```python
from build123d import *

# Parameters (mm, degrees)
F0_R     = 6.35
F1_DEPTH = 3.175


with BuildPart() as f1:
    # F0 (on Front) → F1 (new body, symmetric)
    with BuildSketch(Plane.XZ):
        with BuildLine():
            ThreePointArc((-17.4334869568, 77.4671706545), (-21.0250628511, 76.5704625087), (-24.5709427988, 75.5073358467))
            ThreePointArc((-24.5709427988, 75.5073358467), (-28.0634202853, 74.2801012289), (-31.4949046301, 72.8914259638))
            ThreePointArc((-31.4949046301, 72.8914259638), (-29.5170408255, 62.9143726492), (-19.6585851248, 60.4114964503))
            ThreePointArc((-19.6585851248, 60.4114964503), (-14.8988685075, 63.8720589464), (-13.081, 69.469))
            ThreePointArc((-13.081, 69.469), (-14.2395846465, 74.0218803116), (-17.4334869568, 77.4671706545))
        make_face()
        with BuildLine():
            ThreePointArc((-24.5709427988, 75.5073358467), (-18.8747057723, 74.6070875222), (-16.256, 69.469))
            ThreePointArc((-16.256, 69.469), (-26.3372942277, 64.3309124778), (-24.5709427988, 75.5073358467))
        make_face(mode=Mode.SUBTRACT)
        with BuildLine():
            ThreePointArc((-31.4949046301, 72.8914259638), (-28.0634202853, 74.2801012289), (-24.5709427988, 75.5073358467))
            ThreePointArc((-24.5709427988, 75.5073358467), (-21.0250628511, 76.5704625087), (-17.4334869568, 77.4671706545))
            ThreePointArc((-17.4334869568, 77.4671706545), (-25.5534143712, 78.5265037137), (-31.4949046301, 72.8914259638))
        make_face()
        with BuildLine():
            ThreePointArc((59.6305906851, 52.4335927744), (24.5319973939, 75.5199980174), (-17.4334869568, 77.4671706545))
            ThreePointArc((-17.4334869568, 77.4671706545), (-14.2395846465, 74.0218803116), (-13.081, 69.469))
            ThreePointArc((-13.081, 69.469), (-14.8988685075, 63.8720589464), (-19.6585851248, 60.4114964503))
            ThreePointArc((-19.6585851248, 60.4114964503), (19.192650723, 60.561134655), (50.8659607408, 38.0613046332))
            ThreePointArc((50.8659607408, 38.0613046332), (50.9228529034, 47.8852145144), (59.6305906851, 52.4335927744))
        make_face()
        with BuildLine():
            ThreePointArc((-19.6585851248, 60.4114964503), (-29.5170408255, 62.9143726492), (-31.4949046301, 72.8914259638))
            ThreePointArc((-31.4949046301, 72.8914259638), (-62.5829136435, 48.8719542947), (-78.3514836066, 12.8892984033))
            ThreePointArc((-78.3514836066, 12.8892984033), (-68.4945244609, 13.5260066408), (-63.373, 5.08))
            ThreePointArc((-63.373, 5.08), (-69.0923257109, -3.6516933183), (-79.3819172084, -1.8974237821))
            ThreePointArc((-79.3819172084, -1.8974237821), (-67.3022929991, -42.1365678923), (-36.3814305576, -70.5796040459))
            ThreePointArc((-36.3814305576, -70.5796040459), (-34.1498428756, -61.0672736312), (-24.7158919074, -58.5246406199))
            ThreePointArc((-24.7158919074, -58.5246406199), (-63.4722358852, 2.6989153756), (-19.6585851248, 60.4114964503))
        make_face()
        with BuildLine():
            ThreePointArc((68.58, 42.926), (65.9907092743, 49.4545191171), (59.6305906851, 52.4335927744))
            ThreePointArc((59.6305906851, 52.4335927744), (64.2293016822, 46.6871053087), (68.276185728, 40.5395049195))
            ThreePointArc((68.276185728, 40.5395049195), (68.5037411611, 41.7231220052), (68.58, 42.926))
        make_face()
        with BuildLine():
            ThreePointArc((68.276185728, 40.5395049195), (64.2293016822, 46.6871053087), (59.6305906851, 52.4335927744))
            ThreePointArc((59.6305906851, 52.4335927744), (50.9228529034, 47.8852145144), (50.8659607408, 38.0613046332))
            ThreePointArc((50.8659607408, 38.0613046332), (51.3882284212, 37.3531638847), (51.9006383071, 36.6378576855))
            ThreePointArc((51.9006383071, 36.6378576855), (61.2626352015, 33.6603660866), (68.276185728, 40.5395049195))
        make_face()
        with Locations((59.055, 42.926)):
            Circle(F0_R, mode=Mode.SUBTRACT)
        with BuildLine():
            ThreePointArc((-63.373, 5.08), (-68.4945244609, 13.5260066408), (-78.3514836066, 12.8892984033))
            ThreePointArc((-78.3514836066, 12.8892984033), (-78.8370586265, 9.4766652265), (-79.1740663586, 6.0461734122))
            ThreePointArc((-79.1740663586, 6.0461734122), (-72.4135009686, 11.4114896106), (-66.548, 5.08))
            ThreePointArc((-66.548, 5.08), (-72.8548244643, -1.2698532167), (-79.2474128734, 4.9936509246))
            ThreePointArc((-79.2474128734, 4.9936509246), (-79.3894691896, 1.5495736457), (-79.3819172084, -1.8974237821))
            ThreePointArc((-79.3819172084, -1.8974237821), (-69.0923257109, -3.6516933183), (-63.373, 5.08))
        make_face()
        with BuildLine():
            ThreePointArc((-79.1740663586, 6.0461734122), (-78.8370586265, 9.4766652265), (-78.3514836066, 12.8892984033))
            ThreePointArc((-78.3514836066, 12.8892984033), (-82.3999562618, 5.7421572308), (-79.3819172084, -1.8974237821))
            ThreePointArc((-79.3819172084, -1.8974237821), (-79.3894691896, 1.5495736457), (-79.2474128734, 4.9936509246))
            ThreePointArc((-79.2474128734, 4.9936509246), (-79.2326375079, 5.5214381539), (-79.1740663586, 6.0461734122))
        make_face()
        with BuildLine():
            ThreePointArc((79.4045905265, 0), (76.5719647362, 21.0195911739), (68.276185728, 40.5395049195))
            ThreePointArc((68.276185728, 40.5395049195), (61.2626352015, 33.6603660866), (51.9006383071, 36.6378576855))
            ThreePointArc((51.9006383071, 36.6378576855), (60.5526018111, 19.2195547913), (63.5295905265, 0))
            ThreePointArc((63.5295905265, 0), (60.5526018111, -19.2195547913), (51.9006383071, -36.6378576855))
            ThreePointArc((51.9006383071, -36.6378576855), (61.2626352015, -33.6603660866), (68.276185728, -40.5395049195))
            ThreePointArc((68.276185728, -40.5395049195), (76.5719647362, -21.0195911739), (79.4045905265, 0))
        make_face()
        with BuildLine():
            ThreePointArc((-22.8093313363, -59.2937035145), (-23.7657227015, -58.9168846507), (-24.7158919074, -58.5246406199))
            ThreePointArc((-24.7158919074, -58.5246406199), (-34.1498428756, -61.0672736312), (-36.3814305576, -70.5796040459))
            ThreePointArc((-36.3814305576, -70.5796040459), (-29.7043860041, -73.6392453031), (-22.7732002069, -76.0688526864))
            ThreePointArc((-22.7732002069, -76.0688526864), (-19.1229764719, -72.5674860284), (-17.78, -67.691))
            ThreePointArc((-17.78, -67.691), (-19.1334986379, -62.7969024847), (-22.8093313363, -59.2937035145))
        make_face()
        with Locations((-27.305, -67.691)):
            Circle(F0_R, mode=Mode.SUBTRACT)
        with BuildLine():
            ThreePointArc((-22.7732002069, -76.0688526864), (-29.7043860041, -73.6392453031), (-36.3814305576, -70.5796040459))
            ThreePointArc((-36.3814305576, -70.5796040459), (-30.8681979815, -76.5244163914), (-22.7732002069, -76.0688526864))
        make_face()
        with BuildLine():
            ThreePointArc((50.8659607408, -38.0613046332), (17.5925354611, -61.0451600745), (-22.8093313363, -59.2937035145))
            ThreePointArc((-22.8093313363, -59.2937035145), (-19.1334986379, -62.7969024847), (-17.78, -67.691))
            ThreePointArc((-17.78, -67.691), (-19.1229764719, -72.5674860284), (-22.7732002069, -76.0688526864))
            ThreePointArc((-22.7732002069, -76.0688526864), (21.892308832, -76.3270319788), (59.6305906851, -52.4335927744))
            ThreePointArc((59.6305906851, -52.4335927744), (50.9228529034, -47.8852145144), (50.8659607408, -38.0613046332))
        make_face()
        with BuildLine():
            ThreePointArc((68.58, -42.926), (68.5037411611, -41.7231220052), (68.276185728, -40.5395049195))
            ThreePointArc((68.276185728, -40.5395049195), (64.2293016822, -46.6871053087), (59.6305906851, -52.4335927744))
            ThreePointArc((59.6305906851, -52.4335927744), (65.9907092743, -49.4545191171), (68.58, -42.926))
        make_face()
        with BuildLine():
            ThreePointArc((59.6305906851, -52.4335927744), (64.2293016822, -46.6871053087), (68.276185728, -40.5395049195))
            ThreePointArc((68.276185728, -40.5395049195), (61.2626352015, -33.6603660866), (51.9006383071, -36.6378576855))
            ThreePointArc((51.9006383071, -36.6378576855), (51.3882284212, -37.3531638847), (50.8659607408, -38.0613046332))
            ThreePointArc((50.8659607408, -38.0613046332), (50.9228529034, -47.8852145144), (59.6305906851, -52.4335927744))
        make_face()
        with Locations((59.055, -42.926)):
            Circle(F0_R, mode=Mode.SUBTRACT)
    extrude(amount=F1_DEPTH, both=True)


solid = f1.part
```
Design review of the part built by this model. Coordinates are the model's own, in mm. Give positions to 0.01 mm unless a question says otherwise; leave off trailing zeros. Loops run counter-clockwise (first coordinate to the right, second up) from the corner with the lowest first, then second, coordinate; pieces in that order, holes last. Notation, with made-up numbers: M 54.5,27.25 L 100.5,27.25 A7 ccw 100.5,35.25 Z; hole C 50.25,43 d11. An arc over 180 degrees is marked long. Return JSON: item names as keys, results as strings. Group by question number.
Item 1: For probe 1 along Z at (x, y) = (64, -2.25); probe 2 along X at (y, z) = (2.25, 50.5); probe 3 along Z at (x, y) = (10, 0.25), list the stretches that pass through material, from the lowest coordinate up.
Item 2: We need section C-C (z = -34.5). Give the boundary of the cut face in (x, y) (3 decimals), and give its area (3 significant figures).
Item 3: We need section B-B (y = -1.75). Give the number of separate pieces and of enclosed holes in the cut face, and give its area (3 significant figures).
Item 4: Insertion check: pin 1 Ø10 at (x, z) = (59.055, 42.926) entering from -Y. The pin has a flat end and moves straight along its axis. Give the tip position at first contact, or say it passes through.
Item 5: Mouldability with a two-part tool opening along X and no side actions: class faces 1 (the flat face through (-25.9, 3.175, -58.4)), 2 (the cylindrical face through (-25.441, -0.044, 78.562)), 3 (the cylindrical face through (-62.24, -0.04, 49.31)) as released by +X, released by -X, zero draft, split by the parting line, or undercut.
Item 6: We need section A-A (x = 14). Give the boundary of the cut face in (y, z) (3 decimals).
Output:
{
 "1": {"probe 1": "z = -51.07 to -46.91, -38.94 to 38.94, 46.91 to 51.07", "probe 2": "x = -61.28 to -38.55, 38.55 to 64.83", "probe 3": "z = -78.77 to -62.74, 62.74 to 78.77"},
 "2": {"outline": "M -71.518,-3.175 L -53.346,-3.175 L -53.346,3.175 L -71.518,3.175 Z; M 53.346,-3.175 L 71.518,-3.175 L 71.518,3.175 L 53.346,3.175 Z", "area": "231 mm^2"},
 "3": {"separate pieces": "1", "enclosed holes": "6", "area": "6,660 mm^2"},
 "4": {"pin 1": "passes through"},
 "5": {"face 1": "zero draft", "face 2": "undercut", "face 3": "released by -X"},
 "6": {"outline": "M -3.175,-78.161 L 3.175,-78.161 L 3.175,-61.968 L -3.175,-61.968 Z; M -3.175,61.968 L 3.175,61.968 L 3.175,78.161 L -3.175,78.161 Z"}
}
